The model under review builds one solid part; all positions refer to its coordinate system, in mm. A direction names the side the tool comes from. Coordinates: 2 decimals unless noted, no trailing zeros. Write each loop counter-clockwise with the first axis right and the second up, starting at its lowest first coordinate (ties: lowest second). Pieces come first, ordered by that corner, then holes. Notation, with made-up numbers: (52, -2.75) -> (80, -2.75) arc R21 cw to (80, 9.25) -> close; hole circle Ø1 at (61, 82.5). An arc over 180 degrees is marked (long way). Put each result on its own line as item: value. Start each with the question number.
from build123d import *

# Parameters (mm, degrees)
BOSS_EXTRUDE1_DEPTH     = 10
SKETCH2_R               = 2.6
CUT_EXTRUDE1_DEPTH      = 142.774468788
BOSS_EXTRUDE3_START     = 10
SKETCH3_W               = 60
SKETCH3_H               = 9
SKETCH3_W_2             = 9
SKETCH3_H_2             = 60
BOSS_EXTRUDE3_DEPTH     = 1.46
CUT_EXTRUDE2_DEPTH      = 142.884923794
CUT_EXTRUDE2_DEPTH_BACK = 142.884923794
SKETCH2_2_R             = 2.6
CHAMFER1_SIZE           = 1.46
SKETCH4_R               = 4.5
CUT_EXTRUDE3_DEPTH      = 5
SKETCH5_W               = 100
SKETCH5_H               = 50
SKETCH5_R               = 11.5
SKETCH5_R_2             = 1.75
BOSS_EXTRUDE4_DEPTH     = 5
BOSS_EXTRUDE5_DEPTH     = 10
BOSS_EXTRUDE6_START     = 100
BOSS_EXTRUDE6_DEPTH     = 10
CUT_EXTRUDE4_DEPTH      = 151
CUT_EXTRUDE4_DEPTH_BACK = 151
SKETCH9_R               = 1.75
CUT_EXTRUDE5_START      = 100
SKETCH11_R              = 3
CUT_EXTRUDE5_DEPTH      = 95
SKETCH12_W              = 5
SKETCH12_H              = 10
SKETCH12_W_2            = 10
SKETCH12_H_2            = 5
CUT_EXTRUDE6_DEPTH      = 5
CHAMFER2_SIZE           = 5


with BuildPart() as part:
    # Sketch1 → Boss-Extrude1 (new body)
    with BuildSketch(Plane.XY):
        Polygon((0, 0), (100, 0), (100, 40), (20, 100), (0, 100), align=None)
    extrude(amount=BOSS_EXTRUDE1_DEPTH)

    # Sketch2 → Cut-Extrude1 (cut, through all)
    with BuildSketch(Plane.XY):
        with Locations((10, 85)):
            Circle(SKETCH2_R)
        with Locations((10, 60)):
            Circle(SKETCH2_R)
        with Locations((85, 30)):
            Circle(SKETCH2_R)
        with Locations((85, 10)):
            Circle(SKETCH2_R)
        with Locations((60, 10)):
            Circle(SKETCH2_R)
        with Locations((60, 30)):
            Circle(SKETCH2_R)
    extrude(amount=CUT_EXTRUDE1_DEPTH, mode=Mode.SUBTRACT)

    # Sketch3 → Boss-Extrude3 (add)
    with BuildSketch(Plane.XY.offset(BOSS_EXTRUDE3_START)):
        with Locations((70, 30)):
            Rectangle(SKETCH3_W, SKETCH3_H)
        with Locations((70, 10)):
            Rectangle(SKETCH3_W, SKETCH3_H)
        with Locations((10, 70)):
            Rectangle(SKETCH3_W_2, SKETCH3_H_2)
    extrude(amount=BOSS_EXTRUDE3_DEPTH)

    # Sketch2<2> → Cut-Extrude2 (cut, two sides: drawn at the far end of the back side and taken through both)
    with BuildSketch(Plane.XY.offset(-CUT_EXTRUDE2_DEPTH_BACK)):
        with Locations((10, 85)):
            Circle(SKETCH2_2_R)
        with Locations((10, 60)):
            Circle(SKETCH2_2_R)
        with Locations((85, 30)):
            Circle(SKETCH2_2_R)
        with Locations((85, 10)):
            Circle(SKETCH2_2_R)
        with Locations((60, 10)):
            Circle(SKETCH2_2_R)
        with Locations((60, 30)):
            Circle(SKETCH2_2_R)
    extrude(amount=CUT_EXTRUDE2_DEPTH + CUT_EXTRUDE2_DEPTH_BACK, mode=Mode.SUBTRACT)

    # Chamfer1
    chamfer1_edges = [part.edges().sort_by_distance(p)[0] for p in [
        (14.5, 70, 11.46),
        (5.5, 70, 11.46),
        (70, 5.5, 11.46),
        (70, 14.5, 11.46),
        (70, 25.5, 11.46),
        (70, 34.5, 11.46),
    ]]
    chamfer(chamfer1_edges, length=CHAMFER1_SIZE - 0.0001)  # a hair under: the kernel refuses the full size

    # Sketch4 → Cut-Extrude3 (cut)
    with BuildSketch(Plane.XY):
        with Locations((10, 85)):
            Circle(SKETCH4_R)
        with Locations((10, 60)):
            Circle(SKETCH4_R)
        with Locations((60, 30)):
            Circle(SKETCH4_R)
        with Locations((85, 30)):
            Circle(SKETCH4_R)
        with Locations((85, 10)):
            Circle(SKETCH4_R)
        with Locations((60, 10)):
            Circle(SKETCH4_R)
    extrude(amount=CUT_EXTRUDE3_DEPTH, mode=Mode.SUBTRACT)

    # Sketch5 → Boss-Extrude4 (add)
    with BuildSketch(Plane(origin=(0, 0, 0), x_dir=(1, 0, 0), z_dir=(0, 1, 0))):
        with Locations((50, 25)):
            Rectangle(SKETCH5_W, SKETCH5_H)
        with Locations(Location((50, 25, 0), (0, 0, 270))):
            Circle(SKETCH5_R, mode=Mode.SUBTRACT)
        with Locations(Location((65.5, 9.5, 0), (0, 0, 270))):
            Circle(SKETCH5_R_2, mode=Mode.SUBTRACT)
        with Locations(Location((34.5, 9.5, 0), (0, 0, 270))):
            Circle(SKETCH5_R_2, mode=Mode.SUBTRACT)
        with Locations(Location((34.5, 40.5, 0), (0, 0, 270))):
            Circle(SKETCH5_R_2, mode=Mode.SUBTRACT)
        with Locations(Location((65.5, 40.5, 0), (0, 0, 270))):
            Circle(SKETCH5_R_2, mode=Mode.SUBTRACT)
    extrude(amount=BOSS_EXTRUDE4_DEPTH)

    # Sketch8 → Boss-Extrude5 (add)
    with BuildSketch(Plane(origin=(0, 0, 0), x_dir=(0, 0, -1), z_dir=(1, 0, 0))):
        Polygon((0, 5), (50, 5), (0, 33.75), align=None)
    extrude(amount=BOSS_EXTRUDE5_DEPTH)

    # Sketch8<2> → Boss-Extrude6 (add)
    with BuildSketch(Plane(origin=(0, 0, 0), x_dir=(0, 0, -1), z_dir=(1, 0, 0)).offset(BOSS_EXTRUDE6_START)):
        Polygon((0, 5), (50, 5), (0, 33.75), align=None)
    extrude(amount=-BOSS_EXTRUDE6_DEPTH)

    # Sketch9 → Cut-Extrude4 (cut, two sides: drawn at the far end of the back side and taken through both)
    with BuildSketch(Plane(origin=(0, 0, 0), x_dir=(1, 0, 0), z_dir=(0, 1, 0)).offset(-CUT_EXTRUDE4_DEPTH_BACK)):
        with Locations(Location((95, 45, 0), (0, 0, 90))):
            Circle(SKETCH9_R)
        with Locations(Location((5, 45, 0), (0, 0, 90))):
            Circle(SKETCH9_R)
        with Locations(Location((5, 5, 0), (0, 0, 90))):
            Circle(SKETCH9_R)
        with Locations(Location((95, 5, 0), (0, 0, 90))):
            Circle(SKETCH9_R)
    extrude(amount=CUT_EXTRUDE4_DEPTH + CUT_EXTRUDE4_DEPTH_BACK, mode=Mode.SUBTRACT)

    # Sketch11 → Cut-Extrude5 (cut)
    with BuildSketch(Plane(origin=(0, 0, 0), x_dir=(1, 0, 0), z_dir=(0, 1, 0)).offset(CUT_EXTRUDE5_START)):
        with Locations(Location((95, 5, 0), (0, 0, 270))):
            Circle(SKETCH11_R)
        with Locations(Location((95, 45, 0), (0, 0, 270))):
            Circle(SKETCH11_R)
        with Locations(Location((5, 5, 0), (0, 0, 270))):
            Circle(SKETCH11_R)
        with Locations(Location((5, 45, 0), (0, 0, 270))):
            Circle(SKETCH11_R)
    extrude(amount=-CUT_EXTRUDE5_DEPTH, mode=Mode.SUBTRACT)

    # Sketch12 → Cut-Extrude6 (cut)
    with BuildSketch(Plane(origin=(0, 0, 0), x_dir=(1, 0, 0), z_dir=(0, 1, 0))):
        with Locations((97.5, 20)):
            Rectangle(SKETCH12_W, SKETCH12_H)
        with Locations((2.5, 20)):
            Rectangle(SKETCH12_W, SKETCH12_H)
        with Locations((50, 47.5)):
            Rectangle(SKETCH12_W_2, SKETCH12_H_2)
    extrude(amount=CUT_EXTRUDE6_DEPTH, mode=Mode.SUBTRACT)

    # Chamfer2
    chamfer2_edges = [part.edges().sort_by_distance(p)[0] for p in [
        (100, 2.5, -50),
        (0, 2.5, -50),
        (60, 70, 0),
        (0, 100, 5),
        (10, 100, 0),
        (0, 66.875, 0),
    ]]
    chamfer(chamfer2_edges, length=CHAMFER2_SIZE)


solid = part.part
1. Consider section B-B on z = -21. State the section outline as (x, y) points (3 decimals), then the cut area to 3 significant figures.
2. Tool access review of faces 4 (the cylindrical face through (93.85, 18.99, -2.23)), 5 (the flat face through (0, 27, -7)), 6 (the flat face through (25, 2, -50)), 7 (the flat face through (10, 13, -14)), 8 (the flat face through (12, 58, 5)): name each direction out of +Z, -Z, +X, -X, +Y, -Y from which nothing blocks a thin tool from reaching the whole face with its end or side.
3. Consider section A-A on z = -40.5. State the section outline as (x, y) points, then the cut area to 3 significant figures.
4. Consider section C-C on x = 85. State how many separate pieces and enclosed holes the cut face has, then the cut area to 3 significant figures.
5. Wall thickness on line 1 (X direction, y = 7.65, z = -45); line 2 (X direction, y = 30, z = 8.5); line 3 (Y direction, x = 85, z = 6.5): over which ranges is each line inside the solid? List them lowest first. Write a range as from..to.
6. The part is to be moulded in two halves that separate along Y. For faces 1 (the cylindrical face through (64.16, 8.28, 2.46)), 2 (the cylindrical face through (3.85, 18.99, -2.23)), 3 (the flat face through (95, 5, -3)), say which applies: released by +Y, released by -Y, zero draft, split by the parting line, or undercut.
7. Insertion check: P1, Ø7, axis at x = 95, z = -45, coming from the +Y side; P2, Ø1.8, axis at x = 95, z = -6.5, coming from the +Y side; P3, Ø10, axis at x = 84, y = 28.5, coming from the -Z side; P4, Ø2, axis at x = 65.5, z = -9.5, coming from the -Y side. Each pin has a flat end and moves straight along its axis. Give the tip position at first contact, or say it passes through.
Output values:
1. outline: (0, 5) -> (5, 5) -> (5, 0) -> (39.218, 0) -> (39.218, 5) -> (10, 5) -> (10, 21.675) -> (0, 21.675) -> close; (60.782, 0) -> (95, 0) -> (95, 5) -> (100, 5) -> (100, 21.675) -> (90, 21.675) -> (90, 5) -> (60.782, 5) -> close
1. area: 676 mm^2
2. face 4: +Y
2. face 5: +Z, -Z, -X, +Y, -Y
2. face 6: -Z, +X, -X, +Y, -Y
2. face 7: -Z, +Y
2. face 8: -Z
3. outline: (0, 0) -> (32.75, 0) -> (32.75, 5) -> (10, 5) -> (10, 10.46) -> (0, 10.46) -> close; (36.25, 0) -> (63.75, 0) -> (63.75, 5) -> (36.25, 5) -> close; (67.25, 0) -> (100, 0) -> (100, 10.46) -> (90, 10.46) -> (90, 5) -> (67.25, 5) -> close
3. area: 574 mm^2
4. separate pieces: 3
4. enclosed holes: 0
4. area: 612 mm^2
5. line 1: x = 0..2, 8..10, 90..92, 98..100
5. line 2: x = 0..57.4, 62.6..82.4, 87.6..100
5. line 3: y = 0..7.4, 12.6..27.4, 32.6..51.25
6. face 1: undercut
6. face 2: zero draft
6. face 3: released by +Y
7. P1: stops at y = 9.89
7. P2: stops at y = 5
7. P3: stops at z = 0
7. P4: passes through
